The model under review builds one solid part; all positions refer to its coordinate system, in mm. Face numbers are marked on the shaded views. A direction names the side the tool comes from. Give positions to 0.01 mm unless a question says otherwise; leave off trailing zeros. Loops run counter-clockwise (first coordinate to the right, second up) from the corner with the lowest first, then second, coordinate; pieces in that order, holes last. Notation, with made-up numbers: (88.25, 33) - (140.25, 33) arc R6 cw to (140.25, 37) - close; hole circle Ø2 at (-21, 16). An arc over 180 degrees is marked (long way). Answer as a JSON object with one key per item and string values.
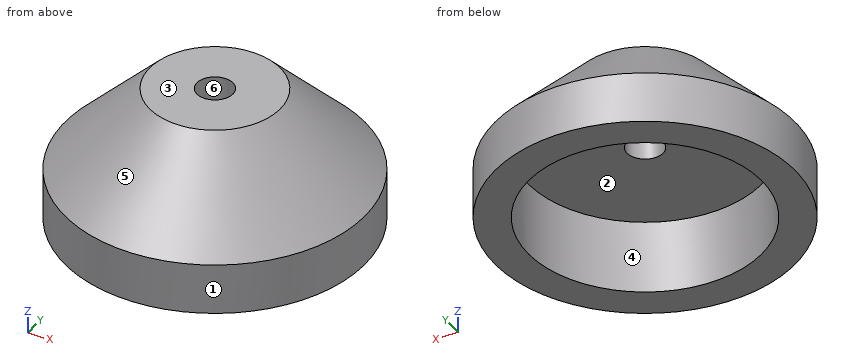
from build123d import *

# Parameters (mm, degrees)
SKETCH1_R                   = 22.5
BOSS_EXTRUDE1_DEPTH         = 20.32
SKETCH2_R                   = 17.5
CUT_EXTRUDE1_DEPTH          = 11
F_1_4_28_TAPPED_HOLE1_D     = 5.4102
F_1_4_28_TAPPED_HOLE1_DEPTH = 9.32
CHAMFER1_SIZE               = 12.7


with BuildPart() as part:
    # Sketch1 → Boss-Extrude1 (new body)
    with BuildSketch(Plane.XY):
        Circle(SKETCH1_R)
    extrude(amount=-BOSS_EXTRUDE1_DEPTH)

    # Sketch2 → Cut-Extrude1 (cut)
    with BuildSketch(Plane(origin=(0, 0, -20.32), x_dir=(-1, 0, 0), z_dir=(0, 0, -1))):
        Circle(SKETCH2_R)
    extrude(amount=-CUT_EXTRUDE1_DEPTH, mode=Mode.SUBTRACT)

    # 1/4-28 Tapped Hole1
    with Locations(Plane.XY):
        with Locations((0, 0)):
            Hole(F_1_4_28_TAPPED_HOLE1_D / 2, depth=F_1_4_28_TAPPED_HOLE1_DEPTH)

    # Chamfer1
    chamfer1_edges = [part.edges().sort_by_distance(p)[0] for p in [
        (-22.5, 0, 0),
    ]]
    chamfer(chamfer1_edges, length=CHAMFER1_SIZE)


solid = part.part
Q1. The part is to be moulded in two halves that separate along Y. For the marked faces 3, 4, 5 and 6, say which applies: +Y half, -Y half, draft (parallel to the pull), parting line (faces both ways), or undercut.
Results:
{"face 3": "draft", "face 4": "undercut", "face 5": "parting line", "face 6": "undercut"}
Q2. Consider section D-D, the plane z = -3.75. State the section outline as (x, y) points.
Results:
{"outline": "circle Ø27.1 at (0, 0); hole circle Ø5.41 at (0, 0)"}
Q3. For the marked faces 1 and 2, list the 3-axis set-ups (+Z, -Z, +X, -X, +Y, -Y) from which the entire face can be reached by the end or side of a thin tool; tool diameter is ignored.
Results:
{"face 1": "+Z, -Z", "face 2": "-Z"}
Q4. Consider section A-A, the plane x = 0. State the section outline as (y, z) points.
Results:
{"outline": "(-22.5, -20.32) - (-17.5, -20.32) - (-17.5, -9.32) - (-2.71, -9.32) - (-2.71, 0) - (-9.8, 0) - (-22.5, -12.7) - close; (2.71, -9.32) - (17.5, -9.32) - (17.5, -20.32) - (22.5, -20.32) - (22.5, -12.7) - (9.8, 0) - (2.71, 0) - close"}
Q5. Clearance check with flat-ended pins moving along their axes: pin 1 Ø12 at (x, z) = (-16, -16) entering from +Y; pin 2 Ø8 at (x, z) = (7.5, -13) entering from +Y; pin 3 Ø3 at (x, y) = (1, -1) entering from -Z. State where each tip first meets the part, or that it passes through.
Results:
{"pin 1": "stops at y = 20.16", "pin 2": "stops at y = 22.23", "pin 3": "stops at z = -9.32"}
Q6. To check wall thickness, follow probe 1 along Y at (x, z) = (0, -16.5); probe 2 along X at (y, z) = (-12, -13.75); probe 3 along X at (y, z) = (8.5, -16). State the ranges of each line that lie inside material, in increasing order. Write a range as [from, to].
Results:
{"probe 1": "y = [-22.5, -17.5], [17.5, 22.5]", "probe 2": "x = [-19.03, -12.74], [12.74, 19.03]", "probe 3": "x = [-20.83, -15.3], [15.3, 20.83]"}
Q7. Consider section C-C, the plane z = -16. State the section outline as (x, y) points.
Results:
{"outline": "circle Ø45 at (0, 0); hole circle Ø35 at (0, 0)"}
